Geometry: see drawing. Coordinates: mm, zero at the bounding-box minimum. A direction names the side the tool comes from. Coordinates: 2 decimals unless noted, no trailing zeros. Write each loop counter-clockwise with the first axis right and the second up, starting at its lowest first coordinate (ties: lowest second). Pieces come first, ordered by that corner, then holes. Notation, with made-up numbers: M -27,58 L -9,58 A8 ccw -9,68 Z; hole C 83.25,79 d2. An arc over 180 degrees is marked long. One line per item, written item: value. Start each with the question number.
Item 1: Cut plane D-D, the plane z = 1.5. Output: boundary loops of the cut face in (x, y), then the cut area to 3 significant figures.
Item 2: Cut plane A-A, the plane y = 3.5. Output: boundary loops of the cut face in (x, z).
Item 3: Pin query (flat end, axial travel): P1, Ø3, axis at x = 5, y = 4, coming from the -Z side. Return the tip coordinate at first contact, or that it passes through.
Item 4: Mould query, pull axis Y, two halves, no side actions, for the marked faces 3, 4 and 5. Classes: released by +Y, released by -Y, zero draft, split by the parting line, or undercut.
Item 5: Set-up query: the marked faces 1 and 2. Return all of +Z, -Z, +X, -X, +Y, -Y with unobstructed straight access to the full face (end or side cutting, diameter ignored); none if empty.
Item 6: Ray query, L1, parallel to Y at x = 3.5, z = 1.2; L2, parallel to Y at x = 3.25, z = 2.2; L3, parallel to X at y = 2.75, z = 0.65. Return the intervals inside material, ascending. Write a range as from..to.
Item 7: Cut plane C-C, the plane z = 0.35. Output: boundary loops of the cut face in (x, y).
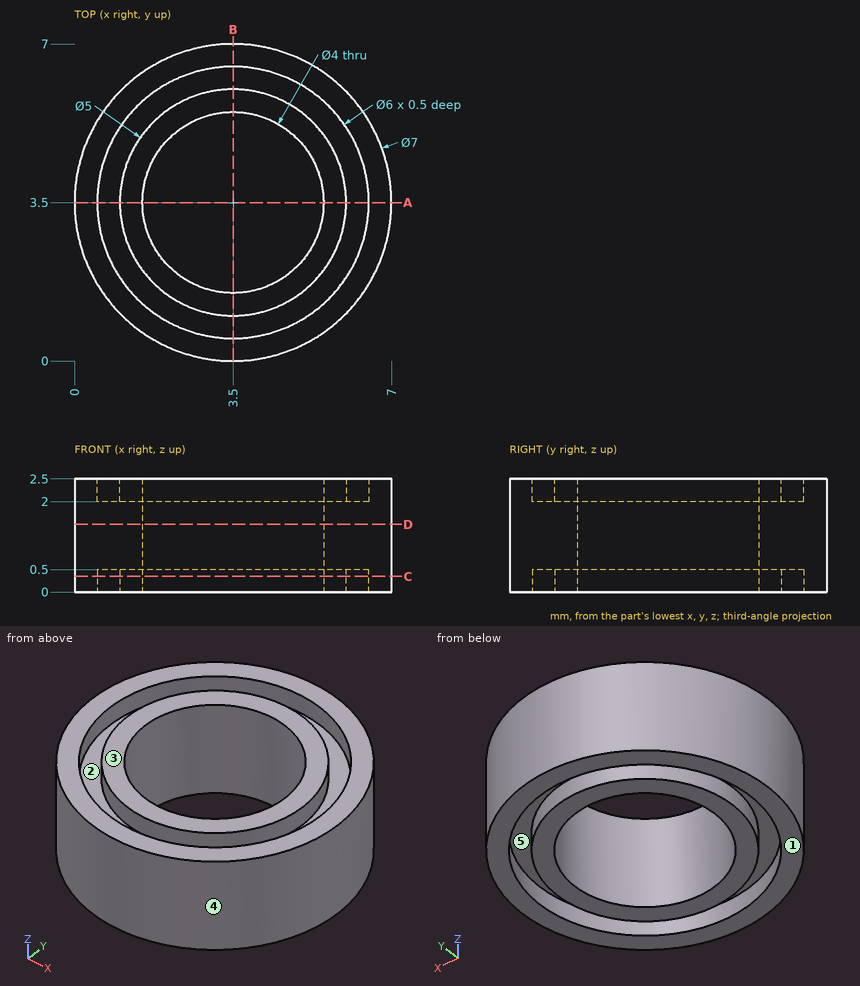
From the geometry:
1. outline: C 3.5,3.5 d7; hole C 3.5,3.5 d4
1. area: 25.9 mm²
2. outline: M 0,0 L 0.5,0 L 0.5,0.5 L 1,0.5 L 1,0 L 1.5,0 L 1.5,2.5 L 1,2.5 L 1,2 L 0.5,2 L 0.5,2.5 L 0,2.5 Z; M 5.5,0 L 6,0 L 6,0.5 L 6.5,0.5 L 6.5,0 L 7,0 L 7,2.5 L 6.5,2.5 L 6.5,2 L 6,2 L 6,2.5 L 5.5,2.5 Z
3. P1: stops at z = 0
4. face 3: zero draft
4. face 4: split by the parting line
4. face 5: undercut
5. face 1: -Z, +X, -X, +Y, -Y
5. face 2: +Z
6. L1: y = 0..1.5, 5.5..7
6. L2: y = 0.01..0.51, 1.01..1.52, 5.48..5.99, 6.49..6.99
6. L3: x = 0.08..1.65, 5.35..6.92
7. outline: C 3.5,3.5 d7; C 3.5,3.5 d5; hole C 3.5,3.5 d6; hole C 3.5,3.5 d4
